Autodesk Inventor part; units mm, degrees
ref_plane "YZ Plane" through (0, 0, 0) normal (1, 0, 0) x (0, 1, 0)
ref_plane "XZ Plane" through (0, 0, 0) normal (0, 1, 0) x (-1, 0, 0)
ref_plane "XY Plane" through (0, 0, 0) normal (0, 0, 1) x (1, 0, 0)
sketch "Skizze1" plane through (0, 0, 0) normal (0, 0, 1) x (1, 0, 0)
  line L0 (0, 0) -> (80, 0)
  line L1 (80, 0) -> (80, 83)
  line L2 (80, 83) -> (0, 83)
  line L3 (0, 83) -> (0, 0)
  line L4 (1.5, 81.5) -> (78.5, 81.5)
  line L5 (78.5, 81.5) -> (78.5, 1.5)
  line L6 (78.5, 1.5) -> (1.5, 1.5)
  line L7 (1.5, 1.5) -> (1.5, 81.5)
  dimension "d0" = 80
  dimension "d1" = 83
  dimension "d2" = 1.5
  dimension "d3" = 1.5
  dimension "d4" = 1.5
  dimension "d5" = 1.5
extrude "Extrusion1" add sketch "Skizze1" along normal blind 2 contours L4 L5 L6 L7
extrude "Extrusion2" add sketch "Skizze1" along normal blind 30
sketch "Skizze2" plane through (0, 0, 2) normal (0, 0, 1) x (1, 0, 0)
  circle A0 centre (22.5, 72.5) radius 3
  circle A1 centre (21, 10.5) radius 3
  line L0 (1.5, 1.5) -> (1.5, 81.5)
  circle A2 centre (22.5, 72.5) radius 2
  circle A3 centre (21, 10.5) radius 2
  circle A4 centre (65.5, 41.5) radius 1
  circle A5 centre (65.5, 41.5) radius 2.5
  line L1 (78.5, 81.5) -> (78.5, 1.5)
  line L2 (78.5, 1.5) -> (1.5, 1.5)
  line L3 (1.5, 81.5) -> (78.5, 81.5)
  line L4 (31.5, 21.5) -> (36.5, 21.5)
  line L5 (36.5, 21.5) -> (36.5, 61.5)
  line L6 (36.5, 61.5) -> (31.5, 61.5)
  line L7 (31.5, 61.5) -> (31.5, 21.5)
  line L8 (6.5, 21.5) -> (11.5, 21.5)
  line L9 (11.5, 21.5) -> (11.5, 61.5)
  line L10 (11.5, 61.5) -> (6.5, 61.5)
  line L11 (6.5, 61.5) -> (6.5, 21.5)
  line L12 (61, 10.5) -> (71, 10.5)
  line L13 (71, 10.5) -> (71, 20.5)
  line L14 (71, 20.5) -> (61, 20.5)
  line L15 (61, 20.5) -> (61, 10.5)
  line L16 (61, 60.5117) -> (71, 60.5117)
  line L17 (71, 60.5117) -> (71, 70.5117)
  line L18 (71, 70.5117) -> (61, 70.5117)
  line L19 (61, 70.5117) -> (61, 60.5117)
  point P0 (0, 0)
  point P1 (71, 65.5117)
  dimension "d11" = 21
  dimension "d12" = 19.5
  dimension "d13" = 4
  dimension "d14" = 4
  dimension "d15" = 6
  dimension "d16" = 6
  dimension "d17" = 2
  dimension "d18" = 5
  dimension "d23" = 13
  dimension "d31" = 62
  dimension "d32" = 9
  dimension "d33" = 9
  dimension "d44" = 5
  dimension "d45" = 40
  dimension "d46" = 30
  dimension "d47" = 20
  dimension "d48" = 20
  dimension "d49" = 5
  dimension "d50" = 40
  dimension "d51" = 20
  dimension "d52" = 5
  dimension "d53" = 10
  dimension "d54" = 10
  dimension "d55" = 10
  dimension "d56" = 10
  dimension "d57" = 7.5
  dimension "d58" = 7.5
extrude "Extrusion3" add sketch "Skizze2" along normal blind 5 contours A0 | A1 | A5 | L7 L6 L5 L4 | L11 L10 L9 L8 | L15 L14 L13 L12 | L19 L18 L17 L16
extrude "Extrusion4" add sketch "Skizze2" along normal blind 10 contours A2 | A3
sketch "Skizze4" plane through (0, 0, 0) normal (0, -1, 0) x (1, 0, 0)
  circle A0 centre (40, 27) radius 1
  line L0 (0, 30) -> (80, 30)
  line L1 (0, 0) -> (0, 30)
  dimension "d34" = 2
  dimension "d35" = 3
  dimension "d36" = 40
extrude "Extrusion6" cut sketch "Skizze4" against normal through all
sketch "Skizze5" plane through (0, 0, 0) normal (0, -1, 0) x (1, 0, 0)
  circle A0 centre (45, 15) radius 3
  line L0 (0, 0) -> (0, 30)
  line L1 (0, 30) -> (80, 30)
  dimension "d39" = 6
  dimension "d40" = 45
  dimension "d41" = 15
extrude "Extrusion7" cut sketch "Skizze5" against normal blind 5
properties part number "Gyrosensor"
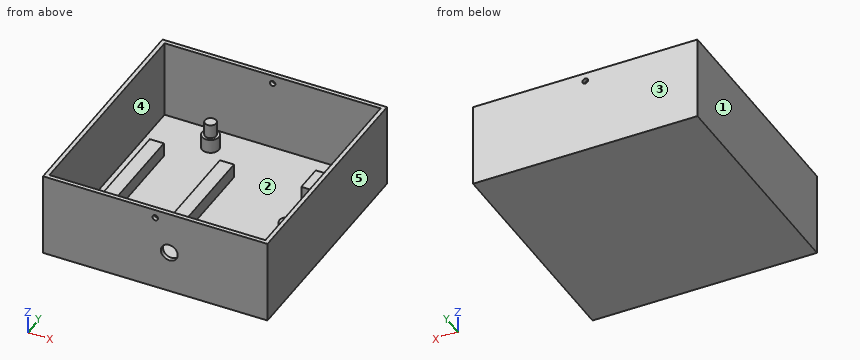
CAD build for the part. Positions are in the model's coordinates, mm. Face numbers are marked on the shaded views. A direction names the side the tool comes from. Coordinates: 2 decimals unless noted, no trailing zeros. Write each loop counter-clockwise with the first axis right and the second up, starting at its lowest first coordinate (ties: lowest second). Pieces come first, ordered by that corner, then holes.
(1) Cut at A-A, the plane z = 8. List the corners of the cut face in (x, y).
(2) Cut at C-C, the plane z = 27. List the corners of the cut face in (x, y).
(3) 3-axis set-ups, long thin cutter, end or side, ignore diameter. For the marked faces 4 and 5: which of +Z, -Z, +X, -X, +Y, -Y reach the whole face in a straight line?
(4) Two-plate mould, pull along Y, no slides. Class the marked faces 1, 2 and 3: +Y half, -Y half, draft (parallel to the pull), parting line (faces both ways), or undercut.
(5) Cut at B-B, the plane x = 45. List the corners of the cut face in (y, z).
(6) Flat gauge pins, fed straight in: pin 1 (8 mm diameter, centred on x = 66, y = 65, fed in from +Z); pin 2 (5 mm diameter, centred on x = 26, y = 67, fed in from +Z); pin 3 (3 mm diameter, centred on x = 22, y = 73.5, fed in from +Z). Where does each tip first touch, or does it go through?
(7) Drill centre lines: probe 1 along Y at (x, z) = (65.5, 3.85); probe 2 along X at (y, z) = (74, 16.5); probe 3 along Y at (x, z) = (48.5, 8.75). Where is each one in solid material? Low to high.
(8) Cut at D-D, the plane y = 68. List the corners of the cut face in (x, z).
Geometry says:
1. outline: (0, 0) - (80, 0) - (80, 83) - (0, 83) - close; circle Ø4 at (21, 10.5); circle Ø4 at (22.5, 72.5); hole (1.5, 1.5) - (78.5, 1.5) - (78.5, 81.5) - (1.5, 81.5) - close
2. outline: (0, 0) - (39, 0) - (39, 1.5) - (1.5, 1.5) - (1.5, 81.5) - (39, 81.5) - (39, 83) - (0, 83) - close; (41, 0) - (80, 0) - (80, 83) - (41, 83) - (41, 81.5) - (78.5, 81.5) - (78.5, 1.5) - (41, 1.5) - close
3. face 4: +Z
3. face 5: +Z, -Z, +X, +Y, -Y
4. face 1: draft
4. face 2: undercut
4. face 3: +Y half
5. outline: (0, 0) - (83, 0) - (83, 30) - (81.5, 30) - (81.5, 2) - (1.5, 2) - (1.5, 12) - (0, 12) - close; (0, 18) - (1.5, 18) - (1.5, 30) - (0, 30) - close
6. pin 1: stops at z = 7
6. pin 2: stops at z = 2
6. pin 3: stops at z = 12
7. probe 1: y = 0 to 1.5, 10.5 to 20.5, 39 to 40.5, 42.5 to 44, 60.51 to 70.51, 81.5 to 83
7. probe 2: x = 0 to 1.5, 78.5 to 80
7. probe 3: y = 0 to 1.5, 81.5 to 83
8. outline: (0, 0) - (80, 0) - (80, 30) - (78.5, 30) - (78.5, 2) - (71, 2) - (71, 7) - (61, 7) - (61, 2) - (1.5, 2) - (1.5, 30) - (0, 30) - close
